The model under review builds one solid part; all positions refer to its coordinate system, in mm. A direction names the side the tool comes from. Coordinates: 2 decimals unless noted, no trailing zeros. Order: outer loops, then holes, each group sorted by start corner. A loop starts at its lowest first (then second) coordinate and runs counter-clockwise, first axis right, second up. Notation, with made-up numbers: (73, -12) -> (93, -12) arc R19 cw to (93, 9) -> close; hole circle Ø6 at (-21, 66). An arc over 180 degrees is marked (long way). Use one line per item in the form item = value.
from build123d import *

# Parameters (mm, degrees)
SKETCH1_R                = 2.54
BOSS_EXTRUDE1_DEPTH      = 1.27
SKETCH2_R                = 3.175
SKETCH2_R_2              = 2.54
BOSS_EXTRUDE2_DEPTH      = 2.54
SKETCH3_R                = 0.9525
CUT_EXTRUDE1_DEPTH       = 0.3175
SCALE1_SCALE             = 1.5
FILLET1_R                = 0.635
SKETCH5_R                = 1.42875
BOSS_EXTRUDE3_DEPTH      = 1.905
BOSS_EXTRUDE4_DEPTH      = 5.08
BOSS_EXTRUDE4_DEPTH_BACK = 5.08
FILLET2_R                = 0.635
BOSS_EXTRUDE5_DEPTH      = 5.461
BOSS_EXTRUDE5_DEPTH_BACK = 5.461
SKETCH9_R                = 4.7625
SKETCH10_R               = 4.2545
SKETCH10_R_2             = 4.0005
CUT_EXTRUDE3_DEPTH       = 0.635
FILLET3_R                = 0.635


with BuildPart() as part:
    # Sketch1 → Boss-Extrude1 (new body)
    with BuildSketch(Plane(origin=(0, 0, 0), x_dir=(1, 0, 0), z_dir=(0, 1, 0))):
        with Locations(Location((0, 0, 0), (0, 0, 270))):
            Circle(SKETCH1_R)
    extrude(amount=BOSS_EXTRUDE1_DEPTH)

    # Sketch2 → Boss-Extrude2 (add)
    with BuildSketch(Plane(origin=(0, 0, 0), x_dir=(1, 0, 0), z_dir=(0, 1, 0))):
        with Locations(Location((0, 0, 0), (0, 0, 270))):
            Circle(SKETCH2_R)
        with Locations(Location((0, 0, 0), (0, 0, 270))):
            Circle(SKETCH2_R_2, mode=Mode.SUBTRACT)
    extrude(amount=BOSS_EXTRUDE2_DEPTH)

    # Sketch3 → Cut-Extrude1 (cut)
    with BuildSketch(Plane.XZ):
        with Locations(Location((0, 0, 0), (0, 0, 270))):
            Circle(SKETCH3_R)
    extrude(amount=-CUT_EXTRUDE1_DEPTH, mode=Mode.SUBTRACT)


with BuildPart() as part_1:
    # Scale1: scaled about (0, 0.984843458, 0)
    add(part.part.scale(SCALE1_SCALE).moved(Location((0, -0.492421729, 0))))

    # Fillet1
    # the kernel refuses this fillet: 0.635 mm, written as the material it takes off along each edge
    with BuildSketch(Plane(origin=(0, -0.492421729, 0), x_dir=(0, 0, -1), z_dir=(-1, 0, 0))) as fillet1_piece_1:
        with BuildLine():
            CenterArc((2.043586106, -0.635), FILLET1_R, 90, 75.522487814)
            Line((1.42875, -0.47625), (1.416453278, -0.473075))
            ThreePointArc((1.416453278, -0.473075), (1.41605, -0.238125), (1.41605, 0))
            Line((1.41605, 0), (1.42875, 0.0127))
            Line((1.42875, 0.0127), (2.043586106, 0.0127))
            Line((2.043586106, 0.0127), (2.043586106, 0))
        make_face()
    revolve(axis=Axis((0, -0.492421729, 0), (0, -1, 0)), mode=Mode.SUBTRACT)

    # Sketch5 → Boss-Extrude3 (add)
    with BuildSketch(Plane.XZ.offset(0.016171729)):
        with Locations(Location((0, 0, 0), (0, 0, 90))):
            Circle(SKETCH5_R)
    extrude(amount=BOSS_EXTRUDE3_DEPTH)

    # Sketch7 → Boss-Extrude4 (add, two sides: drawn at the far end of the back side and taken through both)
    with BuildSketch(Plane.XY.offset(-BOSS_EXTRUDE4_DEPTH_BACK)):
        with BuildLine():
            Line((5.08, -3.826171729), (2.8575, -3.826171729))
            ThreePointArc((2.8575, -3.826171729), (-0.863775136, -2.952658223), (-4.028623369, -5.096171729))
            Line((-4.028623369, -5.096171729), (-5.819871133, -5.096171729))
            ThreePointArc((-5.819871133, -5.096171729), (-0.734899533, -1.328840861), (5.08, -3.826171729))
        make_face()
    extrude(amount=BOSS_EXTRUDE4_DEPTH + BOSS_EXTRUDE4_DEPTH_BACK)

    # Fillet2
    fillet2_edges = [part_1.edges().sort_by_distance(p)[0] for p in [
        (-5.819871133, -5.096171729, 0),
        (5.08, -3.826171729, 0),
        (2.8575, -3.826171729, 0),
        (-4.028623369, -5.096171729, 0),
    ]]
    fillet(fillet2_edges, radius=FILLET2_R)

    # Sketch9 → Boss-Extrude5 (add, two sides: drawn at the far end of the back side and taken through both)
    with BuildSketch(Plane.XY.offset(-BOSS_EXTRUDE5_DEPTH_BACK)):
        with Locations((0, -7.636171729)):
            Circle(SKETCH9_R)
    extrude(amount=BOSS_EXTRUDE5_DEPTH + BOSS_EXTRUDE5_DEPTH_BACK)

    # Sketch10 → Cut-Extrude3 (cut)
    with BuildSketch(Plane(origin=(0, 0, -5.461), x_dir=(-1, 0, 0), z_dir=(0, 0, -1))):
        with Locations((0, -7.636171729)):
            Circle(SKETCH10_R)
        with Locations((0, -7.636171729)):
            Circle(SKETCH10_R_2, mode=Mode.SUBTRACT)
    cut_extrude3 = extrude(amount=-CUT_EXTRUDE3_DEPTH, mode=Mode.SUBTRACT)

    # Mirror1: Cut-Extrude3 across plane
    add(cut_extrude3.mirror(Plane.XY), mode=Mode.SUBTRACT)

    # Fillet3
    # the kernel refuses this fillet: 0.635 mm, written as the material it takes off along each edge
    with BuildSketch(Plane(origin=(3.592102448, -3.826171729, 5.08), x_dir=(0, 1, 0), z_dir=(-1, 0, 0))) as fillet3_piece_1_section:
        with BuildLine():
            CenterArc((FILLET3_R, FILLET3_R), FILLET3_R, 180, 90)
            Line((0, FILLET3_R), (0, 0))
            Line((0, 0), (FILLET3_R, 0))
        make_face()
    fillet3_piece_1 = extrude(amount=2.117743332, mode=Mode.PRIVATE)
    fillet3_piece_1 = fillet3_piece_1 - Plane(origin=(0, -7.636171729, 5.008990652), x_dir=(1, 0, 0), z_dir=(0, 0, -1)) * Cylinder(4.7625, 7, mode=Mode.PRIVATE)
    add(fillet3_piece_1, mode=Mode.SUBTRACT)
    with BuildSketch(Plane(origin=(3.592102448, -3.191171729, 5.08), x_dir=(0.6285393610547108, 0.7777777777777762, 0), z_dir=(-0.7777777777777762, 0.6285393610547108, 0))) as fillet3_piece_2:
        with BuildLine():
            CenterArc((0.635 - FILLET3_R, FILLET3_R), FILLET3_R, 270, 90)
            Line((0.635, FILLET3_R), (0.635, 0))
            Line((0.635, 0), (0.635 - FILLET3_R, 0))
        make_face()
    revolve(axis=Axis((3.592102448, -3.191171729, 5.08), (0, 0, -1)), revolution_arc=141.057558731, mode=Mode.SUBTRACT)
    with BuildSketch(Plane(origin=(-2.777403349, -5.096171729, 5.08), x_dir=(0, 1, 0), z_dir=(-1, 0, 0))) as fillet3_piece_3_section:
        with BuildLine():
            CenterArc((FILLET3_R, FILLET3_R), FILLET3_R, 180, 90)
            Line((0, FILLET3_R), (0, 0))
            Line((0, 0), (FILLET3_R, 0))
        make_face()
    fillet3_piece_3 = extrude(amount=1.974501532, mode=Mode.PRIVATE)
    fillet3_piece_3 = fillet3_piece_3 - Plane(origin=(0, -7.636171729, 4.983808313), x_dir=(1, 0, 0), z_dir=(0, 0, -1)) * Cylinder(4.7625, 7, mode=Mode.PRIVATE)
    add(fillet3_piece_3, mode=Mode.SUBTRACT)
    with BuildSketch(Plane(origin=(-4.751904881, -4.461171729, 5.08), x_dir=(-0.8314794192830989, 0.5555555555555544, 0), z_dir=(0.5555555555555544, 0.8314794192830989, 0))) as fillet3_piece_4:
        with BuildLine():
            CenterArc((0.635 - FILLET3_R, -FILLET3_R), FILLET3_R, 0, 90)
            Line((0.635, -FILLET3_R), (0.635, 0))
            Line((0.635, 0), (0.635 - FILLET3_R, 0))
        make_face()
    revolve(axis=Axis((-4.751904881, -4.461171729, 5.08), (0, 0, 1)), revolution_arc=123.748988596, mode=Mode.SUBTRACT)
    with BuildSketch(Plane(origin=(3.592102448, -3.826171729, -5.08), x_dir=(0, 1, 0), z_dir=(-1, 0, 0))) as fillet3_piece_5_section:
        with BuildLine():
            CenterArc((FILLET3_R, -FILLET3_R), FILLET3_R, 90, 90)
            Line((0, -FILLET3_R), (0, 0))
            Line((0, 0), (FILLET3_R, 0))
        make_face()
    fillet3_piece_5 = extrude(amount=2.117743332, mode=Mode.PRIVATE)
    fillet3_piece_5 = fillet3_piece_5 - Plane(origin=(0, -7.636171729, -5.008990652), x_dir=(1, 0, 0), z_dir=(0, 0, -1)) * Cylinder(4.7625, 7, mode=Mode.PRIVATE)
    add(fillet3_piece_5, mode=Mode.SUBTRACT)
    with BuildSketch(Plane(origin=(3.592102448, -3.191171729, -5.08), x_dir=(0.6285393610547108, 0.7777777777777762, 0), z_dir=(-0.7777777777777762, 0.6285393610547108, 0))) as fillet3_piece_6:
        with BuildLine():
            CenterArc((0.635 - FILLET3_R, -FILLET3_R), FILLET3_R, 0, 90)
            Line((0.635 - FILLET3_R, 0), (0.635, 0))
            Line((0.635, 0), (0.635, -FILLET3_R))
        make_face()
    revolve(axis=Axis((3.592102448, -3.191171729, -5.08), (0, 0, -1)), revolution_arc=141.057558731, mode=Mode.SUBTRACT)
    with BuildSketch(Plane(origin=(-2.777403349, -5.096171729, -5.08), x_dir=(0, 1, 0), z_dir=(-1, 0, 0))) as fillet3_piece_7_section:
        with BuildLine():
            CenterArc((FILLET3_R, -FILLET3_R), FILLET3_R, 90, 90)
            Line((0, -FILLET3_R), (0, 0))
            Line((0, 0), (FILLET3_R, 0))
        make_face()
    fillet3_piece_7 = extrude(amount=1.974501532, mode=Mode.PRIVATE)
    fillet3_piece_7 = fillet3_piece_7 - Plane(origin=(0, -7.636171729, -4.983808313), x_dir=(1, 0, 0), z_dir=(0, 0, -1)) * Cylinder(4.7625, 7, mode=Mode.PRIVATE)
    add(fillet3_piece_7, mode=Mode.SUBTRACT)
    with BuildSketch(Plane(origin=(-4.751904881, -4.461171729, -5.08), x_dir=(-0.8314794192830989, 0.5555555555555544, 0), z_dir=(0.5555555555555544, 0.8314794192830989, 0))) as fillet3_piece_8:
        with BuildLine():
            CenterArc((0.635 - FILLET3_R, FILLET3_R), FILLET3_R, 270, 90)
            Line((0.635 - FILLET3_R, 0), (0.635, 0))
            Line((0.635, 0), (0.635, FILLET3_R))
        make_face()
    revolve(axis=Axis((-4.751904881, -4.461171729, -5.08), (0, 0, 1)), revolution_arc=123.748988596, mode=Mode.SUBTRACT)
    with BuildSketch(Plane(origin=(0, -7.636171729, 5.08), x_dir=(-0.8314794192830981, 0.5555555555555554, 0), z_dir=(-0.5555555555555554, -0.8314794192830981, 0))) as fillet3_piece_9:
        with BuildLine():
            CenterArc((6.35 - FILLET3_R, FILLET3_R), FILLET3_R, 270, 90)
            Line((6.35 - FILLET3_R, 0), (6.35, 0))
            Line((6.35, 0), (6.35, FILLET3_R))
        make_face()
    revolve(axis=Axis((0, -7.636171729, 5.08), (0, 0, -1)), revolution_arc=95.193452673, mode=Mode.SUBTRACT)
    with BuildSketch(Plane(origin=(0, -7.636171729, -5.08), x_dir=(-0.8314794192830981, 0.5555555555555554, 0), z_dir=(-0.5555555555555554, -0.8314794192830981, 0))) as fillet3_piece_10:
        with BuildLine():
            CenterArc((6.35 - FILLET3_R, -FILLET3_R), FILLET3_R, 0, 90)
            Line((6.35 - FILLET3_R, 0), (6.35, 0))
            Line((6.35, 0), (6.35, -FILLET3_R))
        make_face()
    revolve(axis=Axis((0, -7.636171729, -5.08), (0, 0, -1)), revolution_arc=95.193452673, mode=Mode.SUBTRACT)


solid = part_1.part
Item 1: We need section C-C (y = -6.5). Write out the cut boundary in (x, z).
Results found:
outline = (-4.62, -5.46) -> (-4.1, -5.46) -> (-4.1, -4.83) -> (-3.84, -4.83) -> (-3.84, -5.46) -> (3.84, -5.46) -> (3.84, -4.83) -> (4.1, -4.83) -> (4.1, -5.46) -> (4.62, -5.46) -> (4.62, 5.46) -> (4.1, 5.46) -> (4.1, 4.83) -> (3.84, 4.83) -> (3.84, 5.46) -> (-3.84, 5.46) -> (-3.84, 4.83) -> (-4.1, 4.83) -> (-4.1, 5.46) -> (-4.62, 5.46) -> close
Item 2: Clearance check with flat-ended pins moving along their axes: pin 1 (5 mm diameter, centred on y = -0.5, z = -4, fed in from +X); pin 2 (4 mm diameter, centred on x = -1.5, z = 0.5, fed in from +Y); pin 3 (1 mm diameter, centred on x = -4, z = 0, fed in from -Y). State where each tip first meets the part, or that it passes through.
Results found:
pin_1 = 4.52
pin_2 = 1.41
pin_3 = -10.87
Item 3: Tool access review of faces 3 (the face through (-2.9, 1.39, -3.78)), 4 (the face through (0.52, -3.67, 5.15)), 5 (the face through (-5.316, -4.752, 0.062)), 6 (the face through (0.554, -3.418, -5.148)), 7 (the face through (-2, -0.492, 1)): name each direction out of +Z, -Z, +X, -X, +Y, -Y from which nothing blocks a thin tool from reaching the whole face with its end or side.
Results found:
face_3 = +Y
face_4 = +Z
face_5 = +Z, -Z, -X
face_6 = -Z
face_7 = none
Item 4: To check wall thickness, follow L1, parallel to Y at x = 0, z = -5.25; L2, parallel to X at y = 2.2, z = 0; L3, parallel to X at y = -6, z = 5.25. State the ranges of each line that lie inside material, in increasing order. Write a range as from..to.
Results found:
L1 = -12.4..-11.89, -11.64..-3.64, -3.38..-2.87
L2 = -4.76..-3.81, 3.81..4.76
L3 = -4.47..-3.93, -3.65..3.65, 3.93..4.47
Item 5: Draft analysis for pull direction Y (two halves, no side actions). For faces 1 (the face through (-1.417, -0.723, -0.186)), 2 (the face through (0, -8, 5.461)), state which applies: released by +Y, released by -Y, zero draft, split by the parting line, or undercut.
Results found:
face_1 = undercut
face_2 = zero draft
